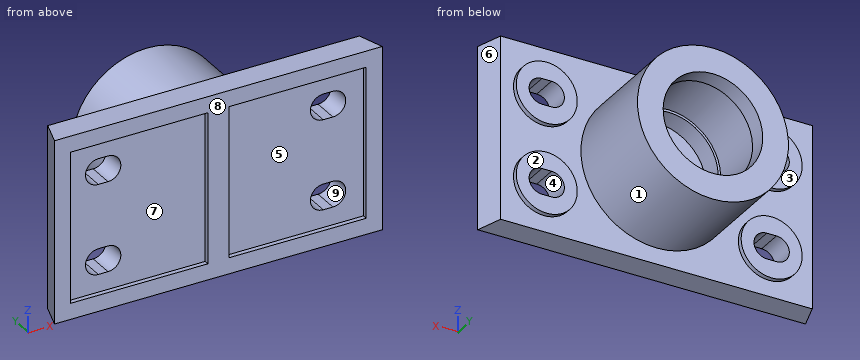
from build123d import *

# Parameters (mm, degrees)
BOSS_EXTRUDE1_DEPTH  = 57
SKETCH2_W            = 85.5
SKETCH2_H            = 94
CUT_EXTRUDE1_DEPTH   = 3
SKETCH4_R            = 47
BOSS_EXTRUDE2_DEPTH  = 61
SKETCH6_R            = 19
BOSS_EXTRUDE4_DEPTH  = 3
CUT_EXTRUDE2_DEPTH   = 20
MIRROR4_COPY_1_DEPTH = 20
SKETCH10_R           = 31
CUT_EXTRUDE3_DEPTH   = 11
SKETCH11_R           = 32.5
CUT_EXTRUDE4_DEPTH   = 37
SKETCH12_R           = 31
CUT_EXTRUDE5_DEPTH   = 13
SKETCH13_R           = 1.5
CUT_EXTRUDE6_DEPTH   = 5


with BuildPart() as part:
    # Sketch1 → Boss-Extrude1 (new body, symmetric)
    with BuildSketch(Plane.XY):
        Polygon((-102, 0), (102, 0), (97, 16), (-97, 16), align=None)
    extrude(amount=BOSS_EXTRUDE1_DEPTH, both=True)

    # Sketch2 → Cut-Extrude1 (cut)
    with BuildSketch(Plane.XZ):
        with Locations((-49.25, 0)):
            Rectangle(SKETCH2_W, SKETCH2_H)
    cut_extrude1 = extrude(amount=-CUT_EXTRUDE1_DEPTH, mode=Mode.SUBTRACT)

    # Mirror1: Cut-Extrude1 across plane
    add(cut_extrude1.mirror(Plane(origin=(0, 0, 0), x_dir=(0, 0, 1), z_dir=(1, 0, 0))), mode=Mode.SUBTRACT)

    # Sketch4 → Boss-Extrude2 (add)
    with BuildSketch(Plane(origin=(0, 16, 0), x_dir=(1, 0, 0), z_dir=(0, 1, 0))):
        with Locations(Location((0, 0, 0), (0, 0, 90))):  # turned: the seam where the file's is
            Circle(SKETCH4_R)
    extrude(amount=BOSS_EXTRUDE2_DEPTH)

    # Sketch6 → Boss-Extrude4 (add)
    with BuildSketch(Plane(origin=(0, 16, 0), x_dir=(1, 0, 0), z_dir=(0, 1, 0))):
        with Locations(Location((70, -28, 0), (0, 0, 90))):  # turned: the seam where the file's is
            Circle(SKETCH6_R)
        with Locations(Location((70, 28, 0), (0, 0, 90))):  # turned: the seam where the file's is
            Circle(SKETCH6_R)
    boss_extrude4 = extrude(amount=BOSS_EXTRUDE4_DEPTH)

    # Sketch9 → Cut-Extrude2 (cut, through all)
    with BuildSketch(Plane(origin=(0, 19, 0), x_dir=(1, 0, 0), z_dir=(0, 1, 0))):
        with BuildLine():
            Line((73, -36), (67, -36))
            ThreePointArc((67, -36), (59, -28), (67, -20))
            Line((67, -20), (73, -20))
            ThreePointArc((73, -20), (81, -28), (73, -36))
        make_face()
    cut_extrude2 = extrude(amount=-CUT_EXTRUDE2_DEPTH, mode=Mode.SUBTRACT)

    # Mirror2: Boss-Extrude4 across plane
    add(boss_extrude4.mirror(Plane(origin=(0, 0, 0), x_dir=(0, 0, 1), z_dir=(1, 0, 0))))

    # Mirror3: Cut-Extrude2 across plane
    add(cut_extrude2.mirror(Plane.XY), mode=Mode.SUBTRACT)

    # Mirror4: Cut-Extrude2 across plane
    add(cut_extrude2.mirror(Plane(origin=(0, 0, 0), x_dir=(0, 0, 1), z_dir=(1, 0, 0))), mode=Mode.SUBTRACT)

    # Mirror4 copy 1 sketch → Mirror4 copy 1 (cut, through all)
    with BuildSketch(Plane(origin=(0, 19, 0), x_dir=(-1, 0, 0), z_dir=(0, 1, 0))):
        with BuildLine():
            Line((73, -36), (67, -36))
            ThreePointArc((67, -36), (59, -28), (67, -20))
            Line((67, -20), (73, -20))
            ThreePointArc((73, -20), (81, -28), (73, -36))
        make_face()
    extrude(amount=-MIRROR4_COPY_1_DEPTH, mode=Mode.SUBTRACT)

    # Sketch10 → Cut-Extrude3 (cut)
    with BuildSketch(Plane(origin=(0, 77, 0), x_dir=(1, 0, 0), z_dir=(0, 1, 0))):
        with Locations(Location((0, 0, 0), (0, 0, 270))):  # turned: the seam where the file's is
            Circle(SKETCH10_R)
    extrude(amount=-CUT_EXTRUDE3_DEPTH, mode=Mode.SUBTRACT)

    # Sketch11 → Cut-Extrude4 (cut)
    with BuildSketch(Plane(origin=(0, 66, 0), x_dir=(1, 0, 0), z_dir=(0, 1, 0))):
        with Locations(Location((0, 0, 0), (0, 0, 270))):  # turned: the seam where the file's is
            Circle(SKETCH11_R)
    extrude(amount=-CUT_EXTRUDE4_DEPTH, mode=Mode.SUBTRACT)

    # Sketch12 → Cut-Extrude5 (cut)
    with BuildSketch(Plane(origin=(0, 29, 0), x_dir=(1, 0, 0), z_dir=(0, 1, 0))):
        with Locations(Location((0, 0, 0), (0, 0, 270))):  # turned: the seam where the file's is
            Circle(SKETCH12_R)
    extrude(amount=-CUT_EXTRUDE5_DEPTH, mode=Mode.SUBTRACT)

    # Sketch13 → Cut-Extrude6 (cut)
    with BuildSketch(Plane(origin=(0, 16, 0), x_dir=(1, 0, 0), z_dir=(0, 1, 0))):
        with Locations(Location((22, 0, 0), (0, 0, 270))):  # turned: the seam where the file's is
            Circle(SKETCH13_R)
    extrude(amount=-CUT_EXTRUDE6_DEPTH, mode=Mode.SUBTRACT)


solid = part.part
Read the model definition and answer for the solid it produces. Units are mm, in the model's axes. Face numbers are marked on the shaded views. A direction names the side the tool comes from. Coordinates: 2 decimals unless noted, no trailing zeros. Loops run counter-clockwise (first coordinate to the right, second up) from the corner with the lowest first, then second, coordinate; pieces in that order, holes last. Notation, with made-up numbers: (88.5, 35.5) -> (147.5, 35.5) arc R17 cw to (147.5, 59.5) -> close; hole circle Ø5 at (5, 51.5). An arc over 180 degrees is marked (long way). Write item = value, one per line. Start each with the question number.
1) The mould has two halves that part along X. Classify the marked faces 6, 7, 8 and 9: pulls with the +X half, pulls with the -X half, needs draft (parallel to the pull), parting line crosses it, or undercut.
2) Given P1, Ø12, axis at y = 60.5, z = 3.5, coming from the -X side; P2, Ø1.5, axis at y = 2, z = 7.5, coming from the +X side; P3, Ø10, axis at y = 60.5, z = 42, coming from the -X side, each flat-ended and moving along its own axis, determine where each tip first touches the part or whether it passes through.
3) The part is cut by section D-D, the plane y = 52. Determine the outline of the cut face in (x, z), plus the area to 3 significant figures.
4) The part is cut by section A-A, the plane x = 70. Determine the outline of the cut face in (y, z).
5) Find the intervals of material crossed by L1, parallel to X at y = 50, z = 0; L2, parallel to X at y = 9, z = 26; L3, parallel to Y at x = -65.5, z = -41, in increasing order. Write a range as from..to.
6) For the marked faces 1, 2, 3, 4 and 5, determine the directions among +Z, -Z, +X, -X, +Y, -Y from which every point of the face is accessible in a straight line to the end or side of a thin tool.
7) The part is cut by section C-C, the plane z = 44. Determine the outline of the cut face in (x, y).
8) The part is cut by section B-B, the plane x = 0. Determine the outline of the cut face in (y, z).
Result:
q1.face_6 = pulls with the +X half
q1.face_7 = undercut
q1.face_8 = needs draft
q1.face_9 = undercut
q2.P1 = -47
q2.P2 = 101.61
q2.P3 = -28.98
q3.outline = circle Ø94 at (0, 0); hole circle Ø65 at (0, 0)
q3.area = 3,620 mm²
q4.outline = (0, -57) -> (16, -57) -> (16, -47) -> (19, -47) -> (19, -36) -> (3, -36) -> (3, -47) -> (0, -47) -> close; (0, 47) -> (3, 47) -> (3, 36) -> (19, 36) -> (19, 47) -> (16, 47) -> (16, 57) -> (0, 57) -> close; (3, -20) -> (19, -20) -> (19, -9) -> (16, -9) -> (16, 9) -> (19, 9) -> (19, 20) -> (3, 20) -> close
q5.L1 = -47..-32.5, 32.5..47
q5.L2 = -99.19..-80.75, -59.25..59.25, 80.75..99.19
q5.L3 = 3..19
q6.face_1 = +Y
q6.face_2 = +Z, -Z, +X, +Y
q6.face_3 = +Z, -Z, -X, +Y
q6.face_4 = +Y, -Y
q6.face_5 = -Y
q7.outline = (-102, 0) -> (-92, 0) -> (-92, 3) -> (-6.5, 3) -> (-6.5, 0) -> (6.5, 0) -> (6.5, 3) -> (92, 3) -> (92, 0) -> (102, 0) -> (97, 16) -> (80.25, 16) -> (80.25, 19) -> (59.75, 19) -> (59.75, 16) -> (16.52, 16) -> (16.52, 77) -> (-16.52, 77) -> (-16.52, 16) -> (-59.75, 16) -> (-59.75, 19) -> (-80.25, 19) -> (-80.25, 16) -> (-97, 16) -> close
q8.outline = (0, -57) -> (16, -57) -> (16, -47) -> (77, -47) -> (77, -31) -> (66, -31) -> (66, -32.5) -> (29, -32.5) -> (29, -31) -> (16, -31) -> (16, 31) -> (29, 31) -> (29, 32.5) -> (66, 32.5) -> (66, 31) -> (77, 31) -> (77, 47) -> (16, 47) -> (16, 57) -> (0, 57) -> close
